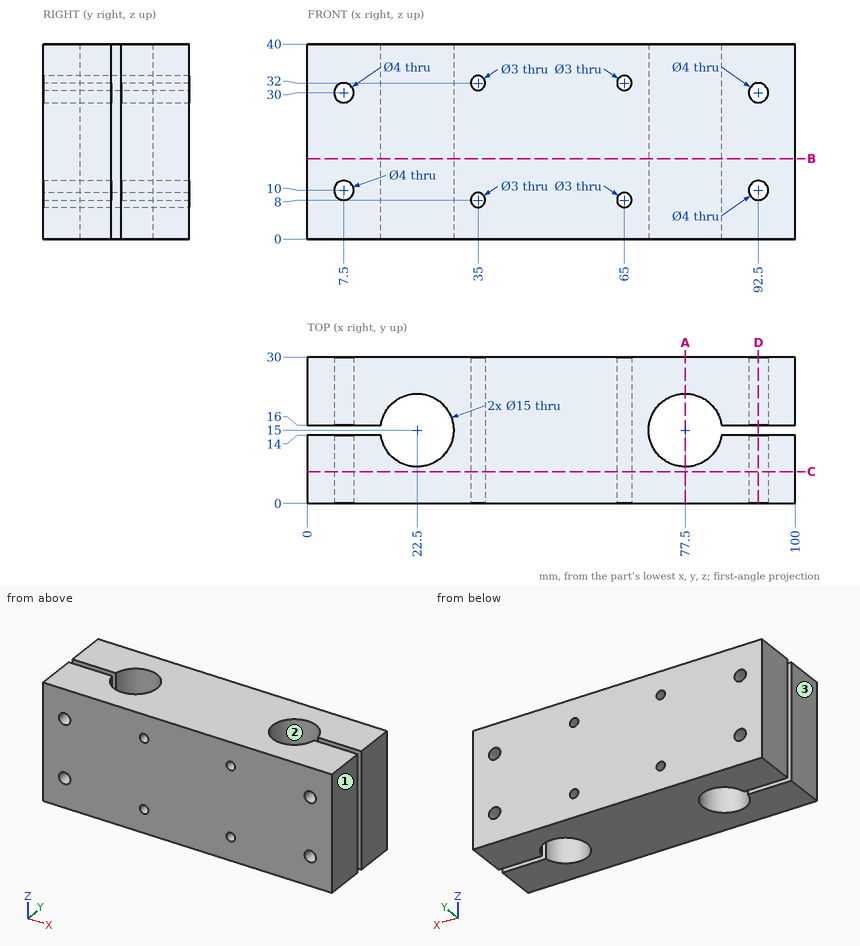
Here's the drawing with two shaded views (mm, measured from the low corner). I have some questions. Coordinates: 2 decimals unless noted, no trailing zeros. Loops run counter-clockwise (first coordinate to the right, second up) from the corner with the lowest first, then second, coordinate; pieces in that order, holes last. Notation, with made-up numbers: (8, 14.25) - (58, 14.25) arc R21 ccw to (58, 40.25) - close; hole circle Ø5 at (-0.5, -0.75). An arc over 180 degrees is marked (long way). Answer as CSV lines item,"result". Start each with the question number.
1) I need wall thicknesses on line 1 (X direction, y = 27.25, z = 30); line 2 (X direction, y = 21, z = 36.5); line 3 (Y direction, x = 89, z = 14). Which ranges of each line are inside material? Lowest first, please. Write a range as from..to.
2) Suppose I cut it at B-B (z = 16.5). Please give me the cut outline in (x, y).
3) For pin 1 (3.5 mm diameter, centred on x = 7.5, z = 30, fed in from -Y); pin 2 (6 mm diameter, centred on x = 64.5, z = 31.5, fed in from -Y), each with a flat end and sliding along its axis, tell me the tip position at first contact or that it passes through.
4) Suppose I cut it at D-D (x = 92.5). Please give me the cut outline in (y, z), plus the area to 3 significant figures.
5) Suppose I cut it at C-C (y = 6.5). Count the separate pieces of the cut face and the enclosed holes in it, plus the area to 3 significant figures.
6) Thinking about a two-plate mould opening in X: for the marked faces 1, 2 and 3, which applies, pulls with the +X half, pulls with the -X half, needs draft (parallel to the pull), parting line crosses it, or undercut?
7) Suppose I cut it at A-A (x = 77.5). Please give me the cut outline in (y, z), plus the area to 3 significant figures.
Check result:
1,line 1,"x = 0..5.5, 9.5..90.5, 94.5..100"
1,line 2,"x = 0..18, 27..73, 82..100"
1,line 3,"y = 0..14, 16..30"
2,outline,"(0, 0) - (100, 0) - (100, 14) - (84.93, 14) arc R7.5 cw (long way) to (84.93, 16) - (100, 16) - (100, 30) - (0, 30) - (0, 16) - (15.07, 16) arc R7.5 cw (long way) to (15.07, 14) - (0, 14) - close"
3,pin 1,"passes through"
3,pin 2,"stops at y = 0"
4,outline,"(0, 0) - (14, 0) - (14, 8) - (0, 8) - close; (0, 12) - (14, 12) - (14, 28) - (0, 28) - close; (0, 32) - (14, 32) - (14, 40) - (0, 40) - close; (16, 0) - (30, 0) - (30, 8) - (16, 8) - close; (16, 12) - (30, 12) - (30, 28) - (16, 28) - close; (16, 32) - (30, 32) - (30, 40) - (16, 40) - close"
4,area,"896 mm²"
5,separate pieces,"1"
5,enclosed holes,"8"
5,area,"3,920 mm²"
6,face 1,"pulls with the +X half"
6,face 2,"undercut"
6,face 3,"pulls with the -X half"
7,outline,"(0, 0) - (7.5, 0) - (7.5, 40) - (0, 40) - close; (22.5, 0) - (30, 0) - (30, 40) - (22.5, 40) - close"
7,area,"600 mm²"
